Input: part model. Units: mm. Frame: model coordinates. Give positions to 0.01 mm unless a question says otherwise; leave off trailing zeros. Order: outer loops, then holes, each group sorted by start corner. A loop starts at its lowest first (then second) coordinate and runs counter-clockwise, first axis right, second up. Notation, with made-up numbers: (77, 1) - (110, 1) arc R15 cw to (110, 22) - close; hole circle Ø9 at (-36, 33). An arc over 180 degrees is marked (long way). Use a Markdown table: item, result.
Autodesk Inventor part; units mm, degrees
sketch "Sketch1" plane through (0, 0, 0) normal (0, 0, 1) x (1, 0, 0)
  circle A0 centre (0, 0) radius 4.1
  circle A1 centre (0, 0) radius 10
  circle A2 centre (0, 8) radius 1.05
  circle A3 centre (-8, 0) radius 1.05
  circle A4 centre (0, -8) radius 1.05
  circle A5 centre (8, 0) radius 1.05
  dimension "d0" = 8.2
  dimension "d7" = 20
  dimension "d33" = 2.1
  dimension "d34" = 8
  dimension "d37" = 360
ref_plane "Work Plane5" through (0, 0, -1) normal (0, 0, -1) x (-1, 0, 0)
sketch "Sketch5" plane through (0, 0, -1) normal (0, 0, -1) x (-1, 0, 0)
  circle A0 centre (0, 0) radius 4.1
  circle A1 centre (0, 0) radius 4.6
  dimension "d30" = 0.5
extrude "Extrusion8" add sketch "Sketch5" along normal blind 10
extrude "Extrusion9" add sketch "Sketch1" along normal mid plane 2
properties part number "porca_roscada_trapezoidal_001" material "Aluminum 6061"
1. Section query A-A (y = -8). Return loops of the section in (x, z).
Response:
| item | result |
|---|---|
| outline | (-6, -1) - (-1.05, -1) - (-1.05, 1) - (-6, 1) - close; (1.05, -1) - (6, -1) - (6, 1) - (1.05, 1) - close |
2. Section query C-C (x = 0). Return loops of the section in (y, z).
Response:
| item | result |
|---|---|
| outline | (-10, -1) - (-9.05, -1) - (-9.05, 1) - (-10, 1) - close; (-6.95, -1) - (-4.6, -1) - (-4.6, -11) - (-4.1, -11) - (-4.1, 1) - (-6.95, 1) - close; (4.1, -11) - (4.6, -11) - (4.6, -1) - (6.95, -1) - (6.95, 1) - (4.1, 1) - close; (9.05, -1) - (10, -1) - (10, 1) - (9.05, 1) - close |
3. Section query D-D (z = -0.75). Return loops of the section in (x, y).
Response:
| item | result |
|---|---|
| outline | circle Ø20 at (0, 0); hole circle Ø2.1 at (-8, 0); hole circle Ø8.2 at (0, 0); hole circle Ø2.1 at (0, -8); hole circle Ø2.1 at (0, 8); hole circle Ø2.1 at (8, 0) |
4. Pin query (flat end, axial travel): pin 1 (1.7 mm diameter, centred on x = 8, y = 0, fed in from +Z); pin 2 (1 mm diameter, centred on x = -3.5, z = -6, fed in from -Y); pin 3 (3.5 mm diameter, centred on x = -8, y = 0, fed in from -Z); pin 4 (5 mm diameter, centred on y = 3.5, z = -6.5, fed in from -X). Return the tip coordinate at first contact, or that it passes through.
Response:
| item | result |
|---|---|
| pin 1 | passes through |
| pin 2 | stops at y = -3.49 |
| pin 3 | stops at z = -1 |
| pin 4 | stops at x = -4.49 |
5. Mould query, pull axis Y, two halves, no side actions, for faces 1 (the face through (4.3, 0.1, 1)), 2 (the face through (-2.17, -9.76, 0.01)), 3 (the face through (0.56, -8.89, -0.01)). Classes: pulls with the +Y half, pulls with the -Y half, needs draft (parallel to the pull), parting line crosses it, or undercut.
Response:
| item | result |
|---|---|
| face 1 | needs draft |
| face 2 | parting line crosses it |
| face 3 | undercut |
6. Material intervals for line 1 along Y through (x, z) = (0, 0.4); line 2 along Y through (x, z) = (0, -6.25); line 3 along Z through (x, y) = (8.5, -3.75), sorted ascending.
Response:
| item | result |
|---|---|
| line 1 | y = -10 to -9.05, -6.95 to -4.1, 4.1 to 6.95, 9.05 to 10 |
| line 2 | y = -4.6 to -4.1, 4.1 to 4.6 |
| line 3 | z = -1 to 1 |
